Can you work these out from the model? Positions are in its coordinate system, mm. A direction names the side the tool comes from. Coordinates: 2 decimals unless noted, no trailing zeros. Order: outer loops, then holes, each group sorted by start corner. A loop starts at its lowest first (then second) coordinate and runs counter-clockwise, first axis right, second up. Notation, with made-up numbers: (-38, -16.5) - (-22, -16.5) arc R26 cw to (-22, 16.5) - close; hole circle Ø5 at (89, 77). An arc over 180 degrees is marked (long way). Use a Markdown table: item, result. Add a question column.
(1) If I drill on L1, parallel to Y at x = -36, z = -5.5; L2, parallel to Y at x = 39.5, z = -244, over which ranges is the centre line in solid material (lowest first)? Write a range as [from, to].
(2) I want a section at B-B (x = 31.5). List the corners of the cut face in (y, z) for me.
(3) I want a section at D-D (x = 0). List the corners of the cut face in (y, z) for me.
(4) On a 3-axis mill with a long thin cutter (end or side, diameter ignored), from which of +Z, -Z, +X, -X, +Y, -Y can I reach the whole of each face in a straight line? I mean faces 4 (the flat face through (1, -44.45, 5)), 5 (the cylindrical face through (-47.18, -46.98, 4.98)). Say none if no direction works.
(5) We'd pull the mould along X, two halves only. Please class faces 1 (the flat face through (-50.8, 1, 5)), 2 (the flat face through (-1, 44.45, 5)), 3 (the cylindrical face through (46.98, -47.18, 4.98)): pulls with the +X half, pulls with the -X half, needs draft (parallel to the pull), parting line crosses it, or undercut.
(6) I want a section at A-A (z = -298.45). List the corners of the cut face in (x, y) for me, and give its area (3 significant figures).
```python
from build123d import *

# Parameters (mm, degrees)
BOSS_EXTRUDE1_DEPTH = 355.6
SKETCH2_R           = 12.7
CUT_EXTRUDE1_DEPTH  = 374.3022368


with BuildPart() as part:
    # Sketch1 → Boss-Extrude1 (new, symmetric)
    with BuildSketch(Plane.XY):
        with BuildLine():
            Line((-38.1, -50.8), (38.1, -50.8))
            ThreePointArc((38.1, -50.8), (47.080256121, -47.080256121), (50.8, -38.1))
            Line((50.8, -38.1), (50.8, 38.1))
            ThreePointArc((50.8, 38.1), (47.080256121, 47.080256121), (38.1, 50.8))
            Line((38.1, 50.8), (-38.1, 50.8))
            ThreePointArc((-38.1, 50.8), (-47.080256121, 47.080256121), (-50.8, 38.1))
            Line((-50.8, 38.1), (-50.8, -38.1))
            ThreePointArc((-50.8, -38.1), (-47.080256121, -47.080256121), (-38.1, -50.8))
        make_face()
        with BuildLine():
            Line((-38.1, 44.45), (38.1, 44.45))
            ThreePointArc((38.1, 44.45), (42.590128061, 42.590128061), (44.45, 38.1))
            Line((44.45, 38.1), (44.45, -38.1))
            ThreePointArc((44.45, -38.1), (42.590128061, -42.590128061), (38.1, -44.45))
            Line((38.1, -44.45), (-38.1, -44.45))
            ThreePointArc((-38.1, -44.45), (-42.590128061, -42.590128061), (-44.45, -38.1))
            Line((-44.45, -38.1), (-44.45, 38.1))
            ThreePointArc((-44.45, 38.1), (-42.590128061, 42.590128061), (-38.1, 44.45))
        make_face(mode=Mode.SUBTRACT)
    extrude(amount=BOSS_EXTRUDE1_DEPTH, both=True)

    # Sketch2 → Cut-Extrude1 (cut, through all)
    with BuildSketch(Plane(origin=(0, 50.8, 0), x_dir=(1, 0, 0), z_dir=(0, 1, 0))):
        with Locations(Location((0, -298.45, 0), (0, 0, 270))):
            Circle(SKETCH2_R)
        with Locations(Location((0, 298.45, 0), (0, 0, 90))):
            Circle(SKETCH2_R)
    extrude(amount=-CUT_EXTRUDE1_DEPTH, mode=Mode.SUBTRACT)


solid = part.part
```
Answers follow:
| question | item | result |
|---|---|---|
| 1 | L1 | y = [-50.8, -44.45], [44.45, 50.8] |
| 1 | L2 | y = [-50.72, -44.29], [44.29, 50.72] |
| 2 | outline | (-50.8, -355.6) - (-44.45, -355.6) - (-44.45, 355.6) - (-50.8, 355.6) - close; (44.45, -355.6) - (50.8, -355.6) - (50.8, 355.6) - (44.45, 355.6) - close |
| 3 | outline | (-50.8, -355.6) - (-44.45, -355.6) - (-44.45, -311.15) - (-50.8, -311.15) - close; (-50.8, -285.75) - (-44.45, -285.75) - (-44.45, 285.75) - (-50.8, 285.75) - close; (-50.8, 311.15) - (-44.45, 311.15) - (-44.45, 355.6) - (-50.8, 355.6) - close; (44.45, -355.6) - (50.8, -355.6) - (50.8, -311.15) - (44.45, -311.15) - close; (44.45, -285.75) - (50.8, -285.75) - (50.8, 285.75) - (44.45, 285.75) - close; (44.45, 311.15) - (50.8, 311.15) - (50.8, 355.6) - (44.45, 355.6) - close |
| 4 | face 4 | +Z, -Z |
| 4 | face 5 | +Z, -Z, -X, -Y |
| 5 | face 1 | pulls with the -X half |
| 5 | face 2 | undercut |
| 5 | face 3 | pulls with the +X half |
| 6 | outline | (-50.8, -38.1) arc R12.7 ccw to (-38.1, -50.8) - (-12.7, -50.8) - (-12.7, -44.45) - (-38.1, -44.45) arc R6.35 cw to (-44.45, -38.1) - (-44.45, 38.1) arc R6.35 cw to (-38.1, 44.45) - (-12.7, 44.45) - (-12.7, 50.8) - (-38.1, 50.8) arc R12.7 ccw to (-50.8, 38.1) - close; (12.7, -50.8) - (38.1, -50.8) arc R12.7 ccw to (50.8, -38.1) - (50.8, 38.1) arc R12.7 ccw to (38.1, 50.8) - (12.7, 50.8) - (12.7, 44.45) - (38.1, 44.45) arc R6.35 cw to (44.45, 38.1) - (44.45, -38.1) arc R6.35 cw to (38.1, -44.45) - (12.7, -44.45) - close |
| 6 | area | 1,990 mm² |
